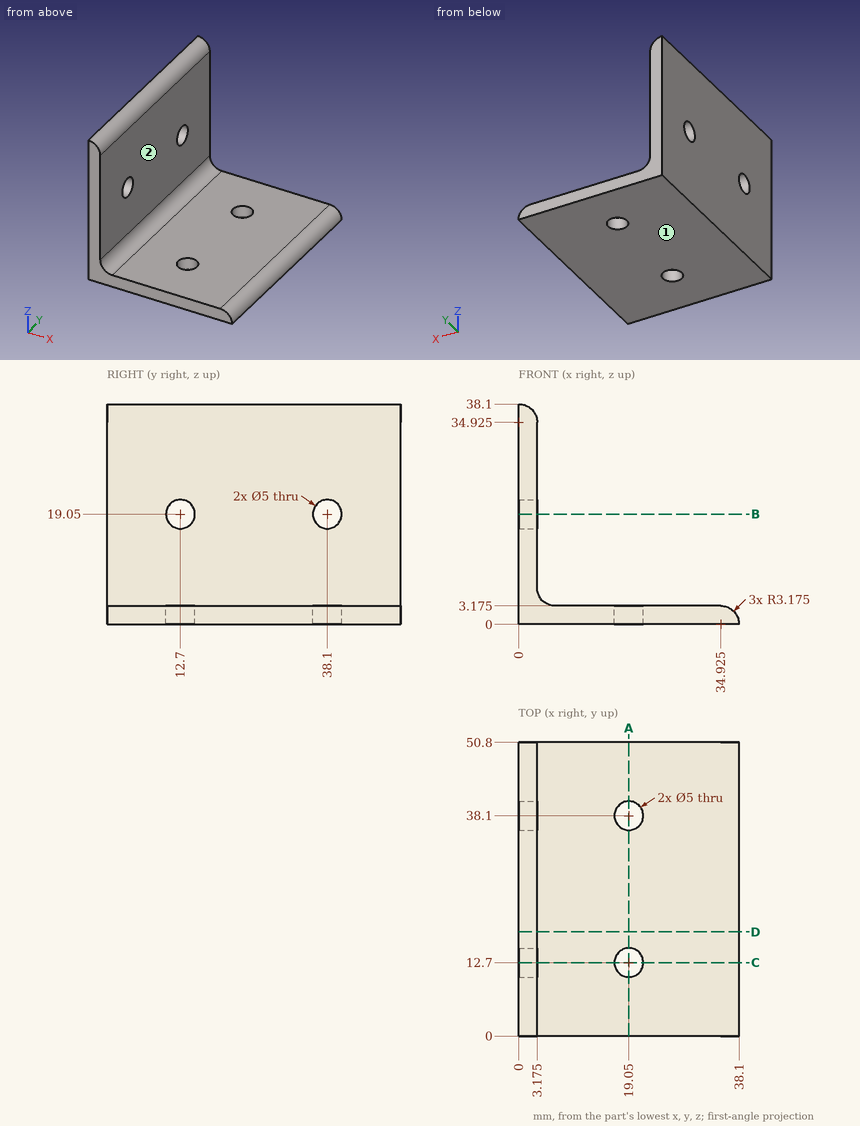
Print and shaded views of the part. All mm, measured from the part's lowest x, y and z. A direction names the side the tool comes from. Round coordinates to 2 decimals unless told otherwise and drop trailing zeros. Write each loop counter-clockwise with the first axis right and the second up, starting at its lowest first coordinate (ties: lowest second). Pieces come first, ordered by that corner, then holes. Notation, with made-up numbers: M 52.5,60.5 L 84.5,60.5 A25 cw 84.5,76.5 Z; hole C 88,48 d3. An arc over 180 degrees is marked long. Use a Markdown table: item, result. Add a question column.
1. Flat gauge pins, fed straight in: P1, Ø8.5, axis at y = 34.5, z = 20.5, coming from the +X side (3 decimals); P2, Ø14.5, axis at x = 15, y = 28, coming from the +Z side (3 decimals). Where does each tip first touch, or does it go through?
2. Slice it at D-D on y = 18. Give the cut face in (x, z) (3 decimals).
3. Slice it at C-C on y = 12.7. Give the cut face in (x, z) (3 decimals), then the cut area to 3 significant figures.
4. Slice it at B-B on z = 19.05. Give the cut face in (x, y) (3 decimals).
5. Drill centre lines: probe 1 along Y at (x, z) = (19, 1); probe 2 along Z at (x, y) = (17.5, 34) (3 decimals). Where is each one in solid material? Low to high.
6. 3-axis set-ups, long thin cutter, end or side, ignore diameter. For the marked faces 1 and 2: which of +Z, -Z, +X, -X, +Y, -Y reach the whole face in a straight line?
7. Slice it at A-A on x = 19.05. Give the cut face in (y, z) (3 decimals).
Reply:
| question | item | result |
|---|---|---|
| 1 | P1 | stops at x = 3.175 |
| 1 | P2 | stops at z = 3.175 |
| 2 | outline | M 0,0 L 38.1,0 A3.175 ccw 34.925,3.175 L 6.35,3.175 A3.175 cw 3.175,6.35 L 3.175,34.925 A3.175 ccw 0,38.1 Z |
| 3 | outline | M 0,0 L 16.55,0 L 16.55,3.175 L 6.35,3.175 A3.175 cw 3.175,6.35 L 3.175,16.55 L 0,16.55 Z; M 0,21.55 L 3.175,21.55 L 3.175,34.925 A3.175 ccw 0,38.1 Z; M 21.55,0 L 38.1,0 A3.175 ccw 34.925,3.175 L 21.55,3.175 Z |
| 3 | area | 198 mm^2 |
| 4 | outline | M 0,0 L 3.175,0 L 3.175,10.2 L 0,10.2 Z; M 0,15.2 L 3.175,15.2 L 3.175,35.6 L 0,35.6 Z; M 0,40.6 L 3.175,40.6 L 3.175,50.8 L 0,50.8 Z |
| 5 | probe 1 | y = 0 to 10.2, 15.2 to 35.6, 40.6 to 50.8 |
| 5 | probe 2 | z = 0 to 3.175 |
| 6 | face 1 | -Z, +X, -X, +Y, -Y |
| 6 | face 2 | +Z, +X, +Y, -Y |
| 7 | outline | M 0,0 L 10.2,0 L 10.2,3.175 L 0,3.175 Z; M 15.2,0 L 35.6,0 L 35.6,3.175 L 15.2,3.175 Z; M 40.6,0 L 50.8,0 L 50.8,3.175 L 40.6,3.175 Z |
